Answer from the drawing. Dimensions are ordinates in mm from the lowest x, y and z of the part. A direction names the side the tool comes from. Round coordinates to 2 decimals unless told otherwise and drop trailing zeros. Write each loop counter-clockwise with the first axis right and the second up, starting at its lowest first coordinate (ties: lowest second). Pieces come first, ordered by that corner, then holes. Notation, with made-up numbers: (39.5, -27.5) - (48.5, -27.5) arc R14 ccw to (48.5, -1.5) - close; hole circle Ø8 at (15, 59.25). An arc over 180 degrees is marked (long way). Use a Markdown table: item, result. Add a question column.
1) A cutting plane is placed at C-C (x = 24.5). Give the vertices of the cut face in (y, z), then the cut area to 3 significant figures.
2) Find the intervals of material crossed by probe 1 along Y at (x, z) = (2.3, 28); probe 2 along Z at (x, y) = (2, 47) (1 decimal); probe 3 along Z at (x, y) = (65, 6.5), in increasing order. Write a range as from..to.
3) A cutting plane is placed at A-A (y = 47.5). Give the vertices of the cut face in (x, z).
4) Each of these flat-tipped pins is pushed along its axis until it touches: P1, Ø5.5, axis at x = 112, y = 12.5, coming from the -Z side; P2, Ø16, axis at x = 76.5, y = 49.5, coming from the +Z side; P3, Ø3, axis at x = 29, z = 42.5, coming from the +Y side; P4, Ø3.5, axis at y = 47.5, z = 11.81, coming from the -X side. Where does it stop, or does it pass through?
5) A tool of negligible diameter and unlimited length cuts with its end or side. For the marked faces 1, 2 and 3, from which of +Z, -Z, +X, -X, +Y, -Y can it reach the whole face along a straight path? Write none if from no direction.
6) A cutting plane is placed at D-D (y = 9). Give the vertices of the cut face in (x, z).
7) A cutting plane is placed at B-B (z = 44). Give the vertices of the cut face in (x, y).
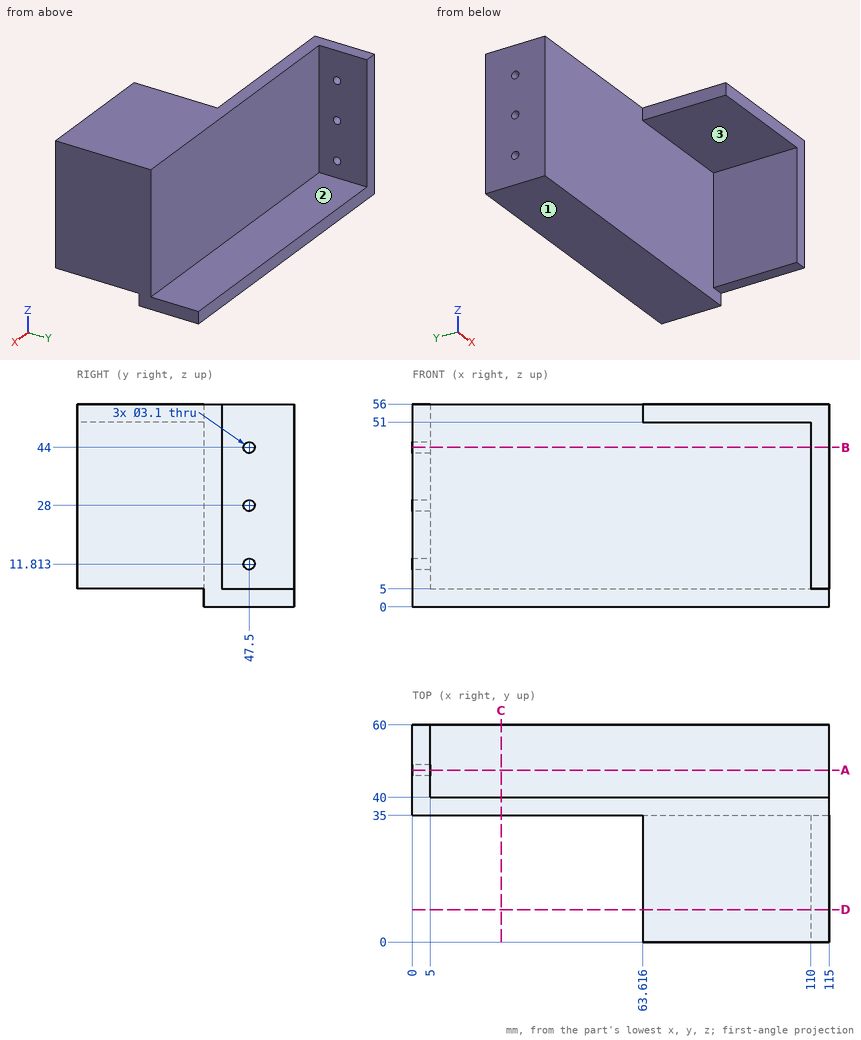
Entries:
| question | item | result |
|---|---|---|
| 1 | outline | (35, 0) - (60, 0) - (60, 5) - (40, 5) - (40, 56) - (35, 56) - close |
| 1 | area | 380 mm² |
| 2 | probe 1 | y = 35..45.95, 49.05..60 |
| 2 | probe 2 | z = 0..10.3, 13.3..26.5, 29.5..42.5, 45.5..56 |
| 2 | probe 3 | z = 51..56 |
| 3 | outline | (0, 0) - (115, 0) - (115, 5) - (5, 5) - (5, 10.26) - (0, 10.26) - close; (0, 13.36) - (5, 13.36) - (5, 26.45) - (0, 26.45) - close; (0, 29.55) - (5, 29.55) - (5, 42.45) - (0, 42.45) - close; (0, 45.55) - (5, 45.55) - (5, 56) - (0, 56) - close |
| 4 | P1 | stops at z = 5 |
| 4 | P2 | stops at z = 5 |
| 4 | P3 | stops at y = 40 |
| 4 | P4 | stops at x = 0 |
| 5 | face 1 | -Z, +X, -X, +Y, -Y |
| 5 | face 2 | +Z, +X, +Y |
| 5 | face 3 | -Z, -X, -Y |
| 6 | outline | (63.62, 51) - (110, 51) - (110, 5) - (115, 5) - (115, 56) - (63.62, 56) - close |
| 7 | outline | (0, 35) - (110, 35) - (110, 0) - (115, 0) - (115, 40) - (5, 40) - (5, 45.95) - (0, 45.95) - close; (0, 49.05) - (5, 49.05) - (5, 60) - (0, 60) - close |
